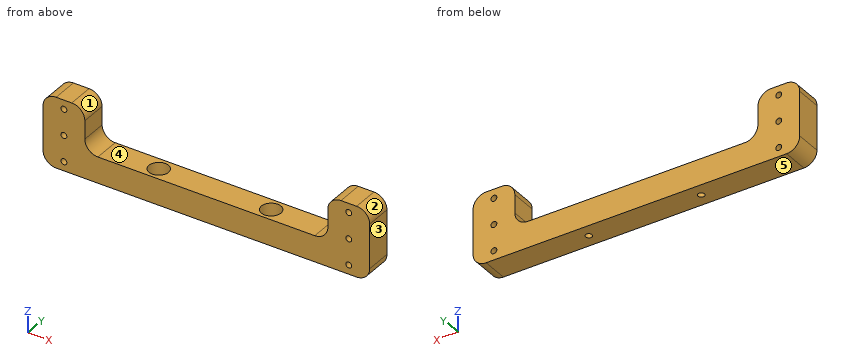
```python
from build123d import *

# Parameters (mm, degrees)
SKETCH1_R           = 2.25
BOSS_EXTRUDE1_DEPTH = 20
SKETCH6_R           = 7.5
CUT_EXTRUDE1_DEPTH  = 16
CUT_EXTRUDE2_REACH  = 6
SKETCH7_R           = 2.5


with BuildPart() as part:
    # Sketch1 → Boss-Extrude1 (new body)
    with BuildSketch(Plane(origin=(0, 0, 0), x_dir=(1, 0, 0), z_dir=(0, 1, 0))):
        with BuildLine():
            Line((115, 20), (-115, 20))
            ThreePointArc((-115, 20), (-122.071067812, 17.071067812), (-125, 10))
            Line((-125, 10), (-125, -24))
            ThreePointArc((-125, -24), (-122.071067812, -31.071067812), (-115, -34))
            Line((-115, -34), (-103, -34))
            ThreePointArc((-103, -34), (-95.928932188, -31.071067812), (-93, -24))
            Line((-93, -24), (-93, -10))
            ThreePointArc((-93, -10), (-90.071067812, -2.928932188), (-83, 0))
            Line((-83, 0), (-30, 0))
            Line((-30, 0), (30, 0))
            Line((30, 0), (83, 0))
            ThreePointArc((83, 0), (90.071067812, -2.928932188), (93, -10))
            Line((93, -10), (93, -24))
            ThreePointArc((93, -24), (95.928932188, -31.071067812), (103, -34))
            Line((103, -34), (115, -34))
            ThreePointArc((115, -34), (122.071067812, -31.071067812), (125, -24))
            Line((125, -24), (125, 10))
            ThreePointArc((125, 10), (122.071067812, 17.071067812), (115, 20))
        make_face()
        with Locations(Location((-109, 13, 0), (0, 0, 270))):  # turned: the seam where the file's is
            Circle(SKETCH1_R, mode=Mode.SUBTRACT)
        with Locations(Location((-109, -7, 0), (0, 0, 270))):  # turned: the seam where the file's is
            Circle(SKETCH1_R, mode=Mode.SUBTRACT)
        with Locations(Location((-109, -27, 0), (0, 0, 270))):  # turned: the seam where the file's is
            Circle(SKETCH1_R, mode=Mode.SUBTRACT)
        with Locations(Location((109, -27, 0), (0, 0, 90))):  # turned: the seam where the file's is
            Circle(SKETCH1_R, mode=Mode.SUBTRACT)
        with Locations(Location((109, -7, 0), (0, 0, 90))):  # turned: the seam where the file's is
            Circle(SKETCH1_R, mode=Mode.SUBTRACT)
        with Locations(Location((109, 13, 0), (0, 0, 90))):  # turned: the seam where the file's is
            Circle(SKETCH1_R, mode=Mode.SUBTRACT)
    extrude(amount=BOSS_EXTRUDE1_DEPTH)

    # Sketch6 → Cut-Extrude1 (cut)
    with BuildSketch(Plane.XY):
        with Locations((-43, 10)):
            Circle(SKETCH6_R)
        with Locations(Location((43, 10, 0), (0, 0, 180))):  # turned: the seam where the file's is
            Circle(SKETCH6_R)
    extrude(amount=-CUT_EXTRUDE1_DEPTH, mode=Mode.SUBTRACT)

    # Sketch7 → Cut-Extrude2 (cut, up to next)
    with BuildSketch(Plane.XY.offset(-16), mode=Mode.PRIVATE) as cut_extrude2_sk1:
        with Locations((-43, 10)):
            Circle(SKETCH7_R)
    cut_extrude2_tool1 = extrude(cut_extrude2_sk1.sketch, amount=-CUT_EXTRUDE2_REACH, mode=Mode.PRIVATE) & part.part
    add(cut_extrude2_tool1.solids().sort_by_distance((-43, 10, -16))[0], mode=Mode.SUBTRACT)
    # Sketch7 → Cut-Extrude2 (cut, up to next)
    with BuildSketch(Plane.XY.offset(-16), mode=Mode.PRIVATE) as cut_extrude2_sk2:
        with Locations((43, 10)):
            Circle(SKETCH7_R)
    cut_extrude2_tool2 = extrude(cut_extrude2_sk2.sketch, amount=-CUT_EXTRUDE2_REACH, mode=Mode.PRIVATE) & part.part
    add(cut_extrude2_tool2.solids().sort_by_distance((43, 10, -16))[0], mode=Mode.SUBTRACT)


solid = part.part
```
The listing builds one solid part. Answer for the finished solid, in the listing's coordinates (mm). Face numbers are marked on the shaded views. A direction names the side the tool comes from. Round coordinates to 2 decimals unless told otherwise and drop trailing zeros. Loops run counter-clockwise (first coordinate to the right, second up) from the corner with the lowest first, then second, coordinate; pieces in that order, holes last.
Q1. Which of the six approach directions +Z, -Z, +X, -X, +Y, -Y give full straight-line access (tool end or side, diameter ignored) to the marked faces 1 and 2?
Q2. For a pull along X with two mould halves and no side action, classify the marked faces 3, 4 and 5 as released by +X, released by -X, zero draft, split by the parting line, or undercut.
Q3. Section B-B, the plane z = 27 is taken. Determine the outline of the cut face in (x, y), then the cut area to 3 significant figures.
Q4. Section D-D, the plane x = 43 is taken. Determine the outline of the cut face in (y, z), then the cut area to 3 significant figures.
Q5. Find the intervals of material crossed by line 1 (X direction, y = 5.75, z = 20); line 2 (X direction, y = 5.5, z = -8.5); line 3 (Y direction, x = 43, z = -19), in increasing order.
Q6. Given pin 1 Ø4 at (x, y) = (43, 10) entering from -Z; pin 2 Ø9 at (x, y) = (43, 10) entering from +Z; pin 3 Ø1 at (y, z) = (4.5, 26.5) entering from -X; pin 4 Ø4 at (y, z) = (2, -13.5) entering from -X, each flat-ended and moving along its own axis, determine where each tip first touches the part or whether it passes through.
Q7. Section A-A, the plane x = -109 is taken. Determine the outline of the cut face in (y, z), then the cut area to 3 significant figures.
Q8. Section C-C, the plane y = 10 is taken. Count the separate pieces of the cut face and the enclosed holes in it, then the cut area to 3 significant figures.
Completed:
1. face 1: +Z, +Y, -Y
1. face 2: +Z, +X, +Y, -Y
2. face 3: released by +X
2. face 4: undercut
2. face 5: zero draft
3. outline: (-124.54, 0) - (-111.25, 0) - (-111.25, 20) - (-124.54, 20) - close; (-106.75, 0) - (-93.46, 0) - (-93.46, 20) - (-106.75, 20) - close; (93.46, 0) - (106.75, 0) - (106.75, 20) - (93.46, 20) - close; (111.25, 0) - (124.54, 0) - (124.54, 20) - (111.25, 20) - close
3. area: 1,060 mm2
4. outline: (0, -20) - (7.5, -20) - (7.5, -16) - (2.5, -16) - (2.5, 0) - (0, 0) - close; (12.5, -20) - (20, -20) - (20, 0) - (17.5, 0) - (17.5, -16) - (12.5, -16) - close
4. area: 140 mm2
5. line 1: x = -125 to -93, 93 to 125
5. line 2: x = -125 to -49, -37 to 37, 49 to 125
5. line 3: y = 0 to 7.5, 12.5 to 20
6. pin 1: passes through
6. pin 2: stops at z = -16
6. pin 3: stops at x = -124.8
6. pin 4: stops at x = -124.89
7. outline: (0, -20) - (20, -20) - (20, -15.25) - (0, -15.25) - close; (0, -10.75) - (20, -10.75) - (20, 4.75) - (0, 4.75) - close; (0, 9.25) - (20, 9.25) - (20, 24.75) - (0, 24.75) - close; (0, 29.25) - (20, 29.25) - (20, 34) - (0, 34) - close
7. area: 810 mm2
8. separate pieces: 3
8. enclosed holes: 6
8. area: 6,470 mm2
